Geometry check sheet. Reference: the model listing, model coordinates, mm. A direction names the side the tool comes from. Coordinates: 2 decimals unless noted, no trailing zeros. Loops run counter-clockwise (first coordinate to the right, second up) from the corner with the lowest first, then second, coordinate; pieces in that order, holes last. Notation, with made-up numbers: M -11.75,78.5 L 43.25,78.5 A16 cw 43.25,109.5 Z; hole C 30.5,-3 d5. An arc over 180 degrees is marked long. Use CSV: the item, a comma, the result in double quotes.
```python
from build123d import *

# Parameters (mm, degrees)
CROQUIS1_W              = 90
CROQUIS1_H              = 25
SALIENTE_EXTRUIR1_DEPTH = 0.9
CROQUIS2_W              = 8
CROQUIS2_H              = 8
CORTAR_EXTRUIR1_DEPTH   = 0.9
CROQUIS3_W              = 79.8
CROQUIS3_H              = 9.8
CROQUIS3_W_2            = 8
CROQUIS3_H_2            = 8
SALIENTE_EXTRUIR2_DEPTH = 20
CROQUIS4_W              = 79.8
CROQUIS4_H              = 9.8
CROQUIS4_R              = 1.5
SALIENTE_EXTRUIR3_DEPTH = 0.9
CROQUIS5_W              = 5
CROQUIS5_H              = 35
CROQUIS5_R              = 1.5
SALIENTE_EXTRUIR4_DEPTH = 2.7


with BuildPart() as part:
    # Croquis1 → Saliente-Extruir1 (new body)
    with BuildSketch(Plane.XY):
        with Locations((-47.428766378, 9.852941176)):
            Rectangle(CROQUIS1_W, CROQUIS1_H)
    extrude(amount=SALIENTE_EXTRUIR1_DEPTH)

    # Croquis2 → Cortar-Extruir1 (cut)
    with BuildSketch(Plane.XY.offset(0.9)):
        with Locations((-82.428766378, 9.852941176)):
            Rectangle(CROQUIS2_W, CROQUIS2_H)
        with Locations((-72.428766378, 9.852941176)):
            Rectangle(CROQUIS2_W, CROQUIS2_H)
        with Locations((-62.428766378, 9.852941176)):
            Rectangle(CROQUIS2_W, CROQUIS2_H)
        with Locations((-52.428766378, 9.852941176)):
            Rectangle(CROQUIS2_W, CROQUIS2_H)
        with Locations((-42.428766378, 9.852941176)):
            Rectangle(CROQUIS2_W, CROQUIS2_H)
        with Locations((-32.428766378, 9.852941176)):
            Rectangle(CROQUIS2_W, CROQUIS2_H)
        with Locations((-22.428766378, 9.852941176)):
            Rectangle(CROQUIS2_W, CROQUIS2_H)
        with Locations((-12.428766378, 9.852941176)):
            Rectangle(CROQUIS2_W, CROQUIS2_H)
    extrude(amount=-CORTAR_EXTRUIR1_DEPTH, mode=Mode.SUBTRACT)

    # Croquis3 → Saliente-Extruir2 (add)
    with BuildSketch(Plane.XY.offset(0.9)):
        with Locations((-47.428766378, 9.852941176)):
            Rectangle(CROQUIS3_W, CROQUIS3_H)
        with Locations((-72.428766378, 9.852941176)):
            Rectangle(CROQUIS3_W_2, CROQUIS3_H_2, mode=Mode.SUBTRACT)
        with Locations((-82.428766378, 9.852941176)):
            Rectangle(CROQUIS3_W_2, CROQUIS3_H_2, mode=Mode.SUBTRACT)
        with Locations((-62.428766378, 9.852941176)):
            Rectangle(CROQUIS3_W_2, CROQUIS3_H_2, mode=Mode.SUBTRACT)
        with Locations((-52.428766378, 9.852941176)):
            Rectangle(CROQUIS3_W_2, CROQUIS3_H_2, mode=Mode.SUBTRACT)
        with Locations((-42.428766378, 9.852941176)):
            Rectangle(CROQUIS3_W_2, CROQUIS3_H_2, mode=Mode.SUBTRACT)
        with Locations((-32.428766378, 9.852941176)):
            Rectangle(CROQUIS3_W_2, CROQUIS3_H_2, mode=Mode.SUBTRACT)
        with Locations((-22.428766378, 9.852941176)):
            Rectangle(CROQUIS3_W_2, CROQUIS3_H_2, mode=Mode.SUBTRACT)
        with Locations((-12.428766378, 9.852941176)):
            Rectangle(CROQUIS3_W_2, CROQUIS3_H_2, mode=Mode.SUBTRACT)
    extrude(amount=SALIENTE_EXTRUIR2_DEPTH)

    # Croquis4 → Saliente-Extruir3 (add)
    with BuildSketch(Plane.XY.offset(20.9)):
        with Locations((-47.428766378, 9.852941176)):
            Rectangle(CROQUIS4_W, CROQUIS4_H)
        with Locations((-82.428766378, 9.852941176)):
            Circle(CROQUIS4_R, mode=Mode.SUBTRACT)
        with Locations((-72.428766378, 9.852941176)):
            Circle(CROQUIS4_R, mode=Mode.SUBTRACT)
        with Locations((-62.428766378, 9.852941176)):
            Circle(CROQUIS4_R, mode=Mode.SUBTRACT)
        with Locations((-52.428766378, 9.852941176)):
            Circle(CROQUIS4_R, mode=Mode.SUBTRACT)
        with Locations((-42.428766378, 9.852941176)):
            Circle(CROQUIS4_R, mode=Mode.SUBTRACT)
        with Locations((-32.428766378, 9.852941176)):
            Circle(CROQUIS4_R, mode=Mode.SUBTRACT)
        with Locations((-22.428766378, 9.852941176)):
            Circle(CROQUIS4_R, mode=Mode.SUBTRACT)
        with Locations((-12.428766378, 9.852941176)):
            Circle(CROQUIS4_R, mode=Mode.SUBTRACT)
    extrude(amount=SALIENTE_EXTRUIR3_DEPTH)

    # Croquis5 → Saliente-Extruir4 (add)
    with BuildSketch(Plane.XZ.offset(-4.952941176)):
        with Locations((-82.428766378, 39.3)):
            Rectangle(CROQUIS5_W, CROQUIS5_H)
        with Locations((-82.428766378, 53.8)):
            Circle(CROQUIS5_R, mode=Mode.SUBTRACT)
        with Locations((-72.428766378, 39.3)):
            Rectangle(CROQUIS5_W, CROQUIS5_H)
        with Locations((-72.428766378, 53.8)):
            Circle(CROQUIS5_R, mode=Mode.SUBTRACT)
        with Locations((-62.428766378, 39.3)):
            Rectangle(CROQUIS5_W, CROQUIS5_H)
        with Locations((-62.428766378, 53.8)):
            Circle(CROQUIS5_R, mode=Mode.SUBTRACT)
        with Locations((-52.428766378, 39.3)):
            Rectangle(CROQUIS5_W, CROQUIS5_H)
        with Locations((-52.428766378, 53.8)):
            Circle(CROQUIS5_R, mode=Mode.SUBTRACT)
        with Locations((-42.428766378, 39.3)):
            Rectangle(CROQUIS5_W, CROQUIS5_H)
        with Locations((-42.428766378, 53.8)):
            Circle(CROQUIS5_R, mode=Mode.SUBTRACT)
        with Locations((-32.428766378, 39.3)):
            Rectangle(CROQUIS5_W, CROQUIS5_H)
        with Locations((-32.428766378, 53.8)):
            Circle(CROQUIS5_R, mode=Mode.SUBTRACT)
        with Locations((-22.428766378, 39.3)):
            Rectangle(CROQUIS5_W, CROQUIS5_H)
        with Locations((-22.428766378, 53.8)):
            Circle(CROQUIS5_R, mode=Mode.SUBTRACT)
        with Locations((-12.428766378, 39.3)):
            Rectangle(CROQUIS5_W, CROQUIS5_H)
        with Locations((-12.428766378, 53.8)):
            Circle(CROQUIS5_R, mode=Mode.SUBTRACT)
    extrude(amount=-SALIENTE_EXTRUIR4_DEPTH)


solid = part.part
```
1. Set-up check for faces 4 (the flat face through (-54.929, 6, 39)), 5 (the flat face through (-68.429, 10, 10)), 6 (the flat face through (-48, 4.953, 16)): record each of +Z, -Z, +X, -X, +Y, -Y from which the full face is reachable in a straight line by a thin tool's end or side.
The answers:
face 4,"+Z, +Y, -Y"
face 5,"-Z"
face 6,"+Z, +X, -X, -Y"
2. Thickness scan on line 1 (Y direction, x = -78.5, z = 10); line 2 (Y direction, x = -12.5, z = 21); line 3 (Y direction, x = -63, z = 23). Record the ranges inside material, lowest first. Write a range as [from, to].
The answers:
line 1,"[4.95, 5.85], [13.85, 14.75]"
line 2,"[4.95, 8.35], [11.35, 14.75]"
line 3,"[4.95, 7.65]"
3. Section check B-B, the plane x = -62. Record the cut outline in (y, z).
The answers:
outline,"M -2.65,0 L 5.85,0 L 5.85,20.9 L 8.42,20.9 L 8.42,21.8 L 7.65,21.8 L 7.65,52.36 L 4.95,52.36 L 4.95,0.9 L -2.65,0.9 Z; M 4.95,55.24 L 7.65,55.24 L 7.65,56.8 L 4.95,56.8 Z; M 11.29,20.9 L 13.85,20.9 L 13.85,0 L 22.35,0 L 22.35,0.9 L 14.75,0.9 L 14.75,21.8 L 11.29,21.8 Z"
4. Release check for a two-part mould opening along Z. For faces 1 (the cylindrical face through (-12.754, 6.284, 52.336)), 2 (the flat face through (-44.929, 6, 39)), 3 (the flat face through (-14.3, 9.9, 20.9)) record: +Z half, -Z half, draft (parallel to the pull), parting line (faces both ways), or undercut.
The answers:
face 1,"undercut"
face 2,"draft"
face 3,"-Z half"
5. Gauge pin test, flat ends, axial feed: P1, Ø9, axis at y = 10.5, z = 14.5, coming from the +X side; P2, Ø6.5, axis at y = 12, z = 12.5, coming from the -X side; P3, Ø6.5, axis at x = -32, z = 9, coming from the -Y side. Record the tip position at first contact, or that the pin passes through.
The answers:
P1,"x = -7.53"
P2,"x = -87.33"
P3,"y = 4.95"
6. Section check A-A, the plane z = 39. Count the separate pieces of the cut face and the enclosed holes in it, plus the area to 3 significant figures.
The answers:
separate pieces,"8"
enclosed holes,"0"
area,"108 mm^2"
